from build123d import *

# Parameters (mm, degrees)
BOSS_EXTRU_1_DEPTH      = 30
BOSS_EXTRU_1_DEPTH_BACK = 15
ESQUISSE1_R             = 3
ESQUISSE1_R_2           = 2.5
ESQUISSE2_R             = 3
ESQUISSE2_R_2           = 2.5
BOSS_EXTRU_2_DEPTH      = 28


with BuildPart() as part:
    # Esquisse1 → Boss.-Extru.1 (new, two sides: drawn at the far end of the back side and taken through both)
    with BuildSketch(Plane.XY.offset(-BOSS_EXTRU_1_DEPTH_BACK)):
        Circle(ESQUISSE1_R)
        Circle(ESQUISSE1_R_2, mode=Mode.SUBTRACT)
    extrude(amount=BOSS_EXTRU_1_DEPTH + BOSS_EXTRU_1_DEPTH_BACK)

    # Esquisse2 → Boss.-Extru.2 (add)
    with BuildSketch(Plane(origin=(0, 0, 0), x_dir=(1, 0, 0), z_dir=(0, 1, 0))):
        Circle(ESQUISSE2_R)
        with Locations(Location((0, 0, 0), (0, 0, 90))):
            Circle(ESQUISSE2_R_2, mode=Mode.SUBTRACT)
    extrude(amount=BOSS_EXTRU_2_DEPTH)


solid = part.part
CAD build for the part. Positions are in the model's coordinates, mm. A direction names the side the tool comes from. Round coordinates to 2 decimals unless told otherwise and drop trailing zeros. Write each loop counter-clockwise with the first axis right and the second up, starting at its lowest first coordinate (ties: lowest second). Pieces come first, ordered by that corner, then holes. Notation, with made-up numbers: M 35,15 L 62,15 A36 ccw 62,54 Z; hole C 83,86 d11. An arc over 180 degrees is marked long. Put each result on its own line as item: value. Start each with the question number.
1) Pin check, flat tips, straight feed: pin 1 Ø1.5 at (x, y) = (2, 9.5) entering from -Z; pin 2 Ø3 at (x, z) = (0, 0) entering from +Y; pin 3 Ø3 at (x, y) = (0, 0) entering from +Z. Stop position of each tip, or through.
2) Saw through at B-B, the plane y = 0.5. Write the cut outline in (x, z), and give its area (3 significant figures).
3) Pull direction Y, two halves, no side cores. Call faces 6 (the cylindrical face through (-0.54, -2.44, 7.18)), 7 (the flat face through (-2, 28, -2)), 8 (the cylindrical face through (-0.65, -2.93, 7.18)): pulls with the +Y half, pulls with the -Y half, needs draft (parallel to the pull), parting line crosses it, or undercut.
4) Saw through at C-C, the plane z = 8. Write the cut outline in (x, y).
5) Saw through at A-A, the plane x = 0. Write the cut outline in (y, z).
6) Drill centre lines: probe 1 along X at (y, z) = (14, 0); probe 2 along Z at (x, y) = (-0.6, 9). Where is each one in solid material? Low to high. Write a range as [from, to].
7) 3-axis set-ups, long thin cutter, end or side, ignore diameter. For faces 1 (the flat face through (-2, 2, -15)), 2 (the flat face through (0, 0, 2.7)), 3 (the cylindrical face through (2.77, 13.8, 1.15)), 4 (the flat face through (-2, 2, 30)), 5 (the cylindrical face through (-0.1, 1, 2.5)): which of +Z, -Z, +X, -X, +Y, -Y reach the whole face in a straight line?
Resolved:
1. pin 1: z = -2.73
1. pin 2: y = 3
1. pin 3: z = 3
2. outline: M -2.96,-15 L -2.45,-15 L -2.45,-1.73 A3 ccw 2.45,-1.73 L 2.45,-15 L 2.96,-15 L 2.96,-0.5 A3 ccw 2.96,0.5 L 2.96,30 L 2.45,30 L 2.45,1.73 A3 ccw -2.45,1.73 L -2.45,30 L -2.96,30 L -2.96,0.5 A3 ccw -2.96,-0.5 Z; hole M -2.45,-0.5 A2.5 ccw 2.45,-0.5 L 2.45,0.5 A2.5 ccw -2.45,0.5 Z
2. area: 51.9 mm²
3. face 6: undercut
3. face 7: pulls with the +Y half
3. face 8: parting line crosses it
4. outline: C 0,0 d6; hole C 0,0 d5
5. outline: M -3,-15 L -2.5,-15 L -2.5,30 L -3,30 Z; M 0,-3 L 2.5,-3 L 2.5,-15 L 3,-15 L 3,-3 L 28,-3 L 28,-2.5 L 3,-2.5 L 3,2.5 L 28,2.5 L 28,3 L 3,3 L 3,30 L 2.5,30 L 2.5,3 L 0,3 L 0,2.5 L 2.5,2.5 L 2.5,-2.5 L 0,-2.5 Z
6. probe 1: [-3, -2.5], [2.5, 3]
6. probe 2: [-2.94, -2.43], [2.43, 2.94]
7. face 1: -Z, +X, -X, +Y, -Y
7. face 2: +Z, -Z
7. face 3: +Y
7. face 4: +Z, +X, -X, +Y, -Y
7. face 5: none
